from build123d import *

# Parameters (mm, degrees)
SKETCH_1_R      = 2
EXTRUDE_1_DEPTH = 3


with BuildPart() as part:
    # 草图1 → 凸台-拉伸1 (new body)
    with BuildSketch(Plane.XY):
        with BuildLine():
            Line((4.993746089, 4.25), (40.006253911, 4.25))
            ThreePointArc((40.006253911, 4.25), (40.667691739, 4.362541391), (41.254690433, 4.6875))
            ThreePointArc((41.254690433, 4.6875), (48.284291264, 5.02129773), (50.795554958, -1.552914271))
            Line((50.795554958, -1.552914271), (51.01040764, -1.767766953))
            Line((51.01040764, -1.767766953), (51.453152975, -2.210512288))
            ThreePointArc((51.453152975, -2.210512288), (58.791461904, -3.267987709), (61.635430691, -10.114948622))
            Line((61.635430691, -10.114948622), (58.192388155, -9.192388155))
            ThreePointArc((58.192388155, -9.192388155), (51.363961031, -6.363961031), (54.192388155, -13.192388155))
            Line((54.192388155, -13.192388155), (55.114948622, -16.635430691))
            ThreePointArc((55.114948622, -16.635430691), (48.267987709, -13.791461904), (47.210512288, -6.453152975))
            Line((47.210512288, -6.453152975), (46.767766953, -6.01040764))
            Line((46.767766953, -6.01040764), (46.552914271, -5.795554958))
            ThreePointArc((46.552914271, -5.795554958), (43.771750949, -5.872938299), (41.254690433, -4.6875))
            ThreePointArc((41.254690433, -4.6875), (40.667691739, -4.362541391), (40.006253911, -4.25))
            Line((40.006253911, -4.25), (4.993746089, -4.25))
            ThreePointArc((4.993746089, -4.25), (4.332308261, -4.362541391), (3.745309567, -4.6875))
            ThreePointArc((3.745309567, -4.6875), (-6, 0), (3.745309567, 4.6875))
            ThreePointArc((3.745309567, 4.6875), (4.332308261, 4.362541391), (4.993746089, 4.25))
        make_face()
        Circle(SKETCH_1_R, mode=Mode.SUBTRACT)
        with Locations(Location((45, 0, 0), (0, 0, 180))):
            Circle(SKETCH_1_R, mode=Mode.SUBTRACT)
    extrude(amount=EXTRUDE_1_DEPTH)


solid = part.part
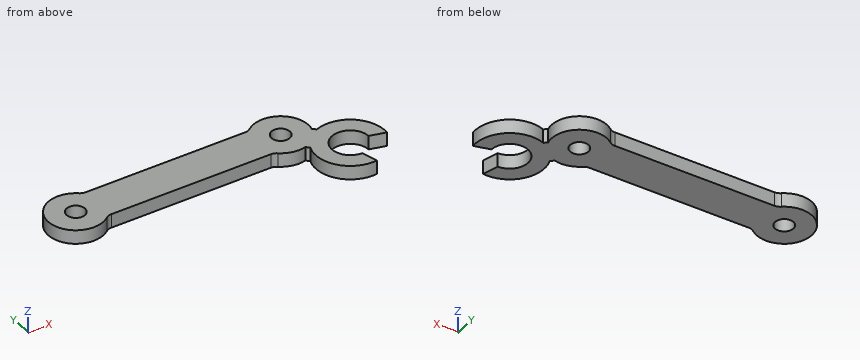
CAD build for the part. Positions are in the model's coordinates, mm. Give positions to 0.01 mm unless a question says otherwise; leave off trailing zeros. Order: outer loops, then holes, each group sorted by start corner. A loop starts at its lowest first (then second) coordinate and runs counter-clockwise, first axis right, second up. Notation, with made-up numbers: (72.25, 80) - (131.25, 80) arc R25 ccw to (131.25, 113) - close; hole circle Ø6 at (54, -19.5). An arc over 180 degrees is marked (long way). Answer in a Markdown table with one row per item.
1. Saw through at D-D, the plane y = -8.25. Give the cut face in (x, z), plus the area to 3 significant figures.
Data:
| item | result |
|---|---|
| outline | (46.75, 0) - (50.3, 0) - (50.3, 3) - (46.75, 3) - close; (58.08, 0) - (61.63, 0) - (61.63, 3) - (58.08, 3) - close |
| area | 21.3 mm² |
2. Saw through at A-A, the plane x = 45. Give the cut face in (y, z), plus the area to 3 significant figures.
Data:
| item | result |
|---|---|
| outline | (-6, 0) - (-2, 0) - (-2, 3) - (-6, 3) - close; (2, 0) - (6, 0) - (6, 3) - (2, 3) - close |
| area | 24.0 mm² |
3. Saw through at C-C, the plane z = 1.5. Give the cut face in (x, y).
Data:
| item | result |
|---|---|
| outline | (3.75, -4.69) arc R2 cw to (4.99, -4.25) - (40.01, -4.25) arc R2 cw to (41.25, -4.69) arc R6 ccw to (46.55, -5.8) - (47.21, -6.45) arc R7.5 ccw to (55.11, -16.64) - (54.19, -13.19) arc R4 cw (long way) to (58.19, -9.19) - (61.64, -10.11) arc R7.5 ccw to (51.45, -2.21) - (50.8, -1.55) arc R6 ccw to (41.25, 4.69) arc R2 cw to (40.01, 4.25) - (4.99, 4.25) arc R2 cw to (3.75, 4.69) arc R6 ccw (long way) to start; hole circle Ø4 at (0, 0); hole circle Ø4 at (45, 0) |
4. Probe probe 1 along X at (y, z) = (-1.5, 0.85); probe 2 along X at (y, z) = (-0.75, 1.45); probe 3 along Y at (x, z) = (45, 2.25). List the from-to ranges inside material, lowest first. Write a range as [from, to].
Data:
| item | result |
|---|---|
| probe 1 | x = [-5.81, -1.32], [1.32, 43.68], [46.32, 50.81] |
| probe 2 | x = [-5.95, -1.85], [1.85, 43.15], [46.85, 50.95] |
| probe 3 | y = [-6, -2], [2, 6] |
5. Flat gauge pins, fed straight in: pin 1 (5 mm diameter, centred on x = 53.5, y = -9.5, fed in from +Z); pin 2 (0.9 mm diameter, centred on x = 19.5, z = 2, fed in from -Y); pin 3 (1.5 mm diameter, centred on x = 19, z = 2, fed in from +Y). Where does each tip first touch, or does it go through?
Data:
| item | result |
|---|---|
| pin 1 | passes through |
| pin 2 | stops at y = -4.25 |
| pin 3 | stops at y = 4.25 |
6. Saw through at B-B, the plane y = 0. Give the cut face in (x, z), plus the area to 3 significant figures.
Data:
| item | result |
|---|---|
| outline | (-6, 0) - (-2, 0) - (-2, 3) - (-6, 3) - close; (2, 0) - (43, 0) - (43, 3) - (2, 3) - close; (47, 0) - (51, 0) - (51, 3) - (47, 3) - close |
| area | 147 mm² |
